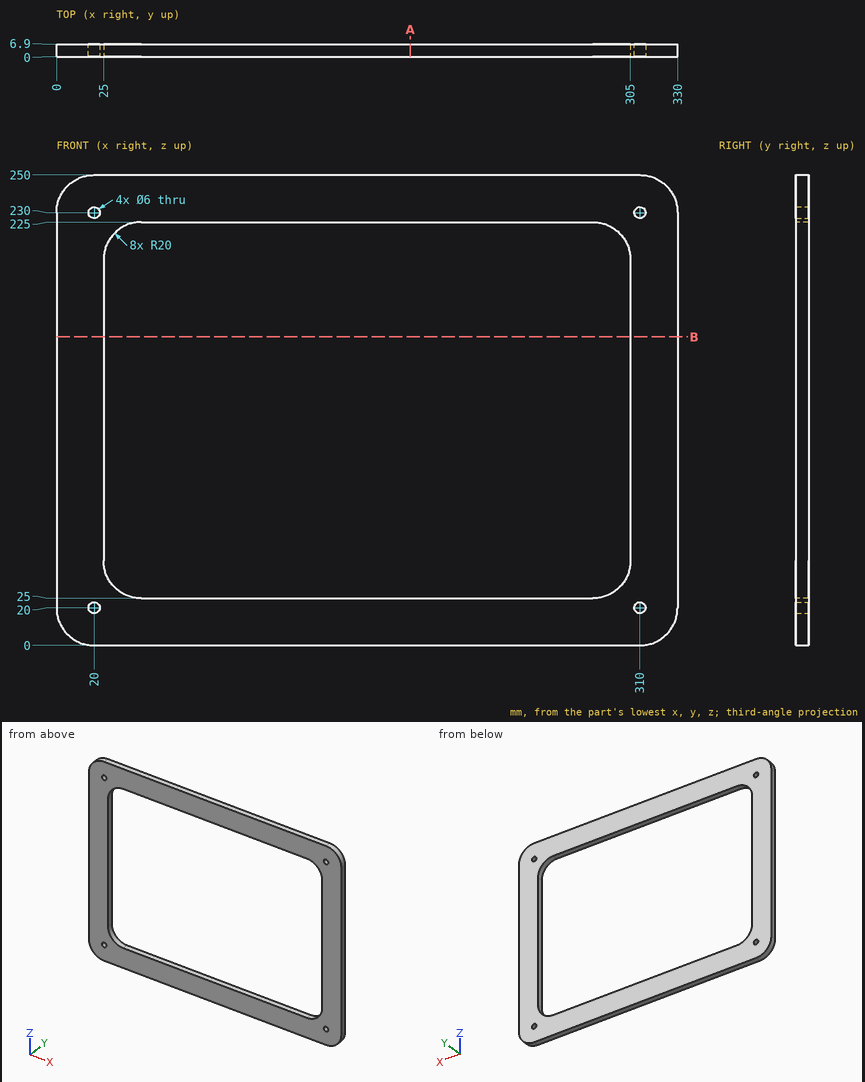
Study the drawing (mm; zero at the part's minimum x, y, z) and answer. Coordinates: 2 decimals unless noted, no trailing zeros. Write each loop counter-clockwise with the first axis right and the second up, starting at its lowest first coordinate (ties: lowest second). Pieces come first, ordered by that corner, then holes. Notation, with made-up numbers: (-37.75, -8.75) - (-1.75, -8.75) arc R17 ccw to (-1.75, 1.25) - close; hole circle Ø2 at (-21.5, 73.5). An arc over 180 degrees is marked (long way). One line per item, written item: value.
1) Find section B-B (z = 164). Give the vertices of the cut face in (x, y).
Geometry check:
outline: (0, 0) - (25, 0) - (25, 6.9) - (0, 6.9) - close; (305, 0) - (330, 0) - (330, 6.9) - (305, 6.9) - close
2) Each of these flat-tipped pins is pushed along its axis until it touches: pin 1 Ø5 at (x, z) = (20, 20) entering from -Y; pin 2 Ø7 at (x, z) = (310, 20) entering from -Y. Where does it stop, or does it pass through?
Geometry check:
pin 1: passes through
pin 2: stops at y = 0
3) Consider line 1 along Z through (x, y) = (310, 4); line 2 along X through (y, z) = (2.75, 230); line 3 along Z through (x, y) = (226.5, 3.75). Determine where each line is inside the solid, lowest interval first. Write a range as from..to.
Geometry check:
line 1: z = 0..17, 23..227, 233..250
line 2: x = 0..17, 23..307, 313..330
line 3: z = 0..25, 225..250
4) Find section A-A (x = 188). Give the vertices of the cut face in (y, z).
Geometry check:
outline: (0, 0) - (6.9, 0) - (6.9, 25) - (0, 25) - close; (0, 225) - (6.9, 225) - (6.9, 250) - (0, 250) - close
